For this review, take the finished solid that the model builds, in its own axes (mm). A direction names the side the tool comes from. Coordinates: 2 decimals unless noted, no trailing zeros. Order: outer loops, then holes, each group sorted by start corner. A loop starts at its lowest first (then second) coordinate and runs counter-clockwise, first axis right, second up.
from build123d import *

# Parameters (mm, degrees)
SKETCH1_W           = 100
SKETCH1_H           = 50
BOSS_EXTRUDE1_DEPTH = 60
CUT_EXTRUDE1_DEPTH  = 50
SKETCH3_R           = 13
CUT_EXTRUDE2_DEPTH  = 50
SKETCH4_R           = 8.30196488
CUT_EXTRUDE3_DEPTH  = 93.736184955
CUT_EXTRUDE4_DEPTH  = 10
SKETCH7_R           = 7.5
CUT_EXTRUDE5_DEPTH  = 10


with BuildPart() as part:
    # Sketch1 → Boss-Extrude1 (new body)
    with BuildSketch(Plane(origin=(0, 0, 0), x_dir=(1, 0, 0), z_dir=(0, 1, 0))):
        Rectangle(SKETCH1_W, SKETCH1_H)
    extrude(amount=BOSS_EXTRUDE1_DEPTH)

    # Sketch2 → Cut-Extrude1 (cut)
    with BuildSketch(Plane(origin=(0, 60, 0), x_dir=(1, 0, 0), z_dir=(0, 1, 0))):
        Polygon((-50, 25), (-36.183650965, 25), (-45, -25), (-50, -25), align=None)
    extrude(amount=-CUT_EXTRUDE1_DEPTH, mode=Mode.SUBTRACT)

    # Sketch3 → Cut-Extrude2 (cut)
    with BuildSketch(Plane(origin=(0, 60, 0), x_dir=(1, 0, 0), z_dir=(0, 1, 0))):
        with Locations(Location((0, 0, 0), (0, 0, 270))):
            Circle(SKETCH3_R)
    extrude(amount=-CUT_EXTRUDE2_DEPTH, mode=Mode.SUBTRACT)

    # Sketch4 → Cut-Extrude3 (cut, through all)
    with BuildSketch(Plane.XY.offset(25)):
        with Locations((25, 30)):
            Circle(SKETCH4_R)
    extrude(amount=-CUT_EXTRUDE3_DEPTH, mode=Mode.SUBTRACT)

    # Sketch6 → Cut-Extrude4 (cut)
    with BuildSketch(Plane(origin=(0, 60, 0), x_dir=(1, 0, 0), z_dir=(0, 1, 0))):
        with BuildLine():
            Line((29, 15), (36, 15))
            ThreePointArc((36, 15), (38.828427125, 13.828427125), (40, 11))
            Line((40, 11), (40, -8))
            ThreePointArc((40, -8), (38.828427125, -10.828427125), (36, -12))
            Line((36, -12), (29, -12))
            ThreePointArc((29, -12), (26.171572875, -10.828427125), (25, -8))
            Line((25, -8), (25, 11))
            ThreePointArc((25, 11), (26.171572875, 13.828427125), (29, 15))
        make_face()
    extrude(amount=-CUT_EXTRUDE4_DEPTH, mode=Mode.SUBTRACT)

    # Sketch7 → Cut-Extrude5 (cut)
    with BuildSketch(Plane.XY.offset(25)):
        with Locations((-20, 30)):
            Circle(SKETCH7_R)
    extrude(amount=-CUT_EXTRUDE5_DEPTH, mode=Mode.SUBTRACT)


solid = part.part
1. Clearance check with flat-ended pins moving along their axes: pin 1 Ø3 at (y, z) = (56.5, -1) entering from -X; pin 2 Ø8 at (x, z) = (-1.5, 0.5) entering from +Y; pin 3 Ø1.5 at (y, z) = (17.5, -17.5) entering from -X; pin 4 Ø15 at (x, y) = (25, 30) entering from -Z. State where each tip first meets the part, or that it passes through.
Answer below:
pin 1: stops at x = -40.68
pin 2: stops at y = 10
pin 3: stops at x = -37.64
pin 4: passes through
2. To check wall thickness, follow L1, parallel to Z at x = -0.5, y = 32; L2, parallel to Y at x = -20, z = 22.5; L3, parallel to X at y = 56, z = 2. State the ranges of each line that lie inside material, in increasing order.
Answer below:
L1: z = -25 to -12.99, 12.99 to 25
L2: y = 0 to 22.5, 37.5 to 60
L3: x = -40.94 to -12.85, 12.85 to 25, 40 to 50
3. Machinability: for faces 1 (the face through (-40.53, 35.35, -0.35)), 2 (the face through (-1, 30, -25)), 3 (the face through (-25.952, 25.436, 20.07)), 4 (the face through (38.859, 55.07, 10.797)), which of the approach directions +Z, -Z, +X, -X, +Y, -Y give a long, thin tool a straight path to every point of the face, cutting with its end or side? Answer none if there is none.
Answer below:
face 1: -Z, -X, +Y
face 2: -Z, +X, -X, +Y, -Y
face 3: +Z
face 4: +Y
4. Take a section at C-C, the plane x = -20. Give the boundary of the cut face in (y, z), plus the area to 3 significant figures.
Answer below:
outline: (0, -25) - (60, -25) - (60, 25) - (37.5, 25) - (37.5, 15) - (22.5, 15) - (22.5, 25) - (0, 25) - close
area: 2,850 mm2
5. Take a section at B-B, the plane y = 52. Give the boundary of the cut face in (x, z), plus the area to 3 significant figures.
Answer below:
outline: (-45, 25) - (-36.18, -25) - (50, -25) - (50, 25) - close; hole circle Ø26 at (0, 0); hole (25, -11) arc R4 ccw to (29, -15) - (36, -15) arc R4 ccw to (40, -11) - (40, 8) arc R4 ccw to (36, 12) - (29, 12) arc R4 ccw to (25, 8) - close
area: 3,610 mm2
6. The part is to be moulded in two halves that separate along Y. For faces 5 (the face through (33, 50, -2)), 6 (the face through (-1, 0, 0)), 7 (the face through (33, 55, 12)), 8 (the face through (-20, 30, 15)), say which applies: +Y half, -Y half, draft (parallel to the pull), parting line (faces both ways), or undercut.
Answer below:
face 5: +Y half
face 6: -Y half
face 7: draft
face 8: undercut
7. Take a section at D-D, the plane z = 20.5. Give the boundary of the cut face in (x, y), plus the area to 3 significant figures.
Answer below:
outline: (-50, 0) - (50, 0) - (50, 60) - (-44.21, 60) - (-44.21, 10) - (-50, 10) - close; hole circle Ø15 at (-20, 30); hole circle Ø16.6 at (25, 30)
area: 5,320 mm2
8. Take a section at A-A, the plane y = 30. Give the boundary of the cut face in (x, z), plus the area to 3 significant figures.
Answer below:
outline: (-45, 25) - (-36.18, -25) - (16.7, -25) - (16.7, 25) - (-12.5, 25) - (-12.5, 15) - (-27.5, 15) - (-27.5, 25) - close; (33.3, -25) - (50, -25) - (50, 25) - (33.3, 25) - close; hole circle Ø26 at (0, 0)
area: 3,020 mm2
